Autodesk Fusion 360 part; units mm, degrees
sketch "Sketch4" plane through (0, 0, 0) normal (0, 0, 1) x (1, 0, 0)
  circle A0 centre (0, 0) radius 12.7
  dimension "d28" = 25.4
extrude "Extrude4" add sketch "Sketch4" along normal blind 25.4
sketch "Sketch5" plane through (0, 0, 25.4) normal (0, 0, 1) x (-1, 0, 0)
  circle A0 centre (0, 0) radius 12.7
  circle A1 centre (0, 0) radius 15.24
extrude "Extrude5" add sketch "Sketch5" along normal blind 5.08 contours A0 | A1
chamfer "Chamfer2" distance 2.54 angle 45 1 edges at (-11.8406, -4.5925, 0)
Verification items for the finished model (mm, model axes). A direction names the side the tool comes from. Coordinates: 2 decimals unless noted, no trailing zeros. Order: outer loops, then holes, each group sorted by start corner. A loop starts at its lowest first (then second) coordinate and runs counter-clockwise, first axis right, second up.
1. Set-up check for faces 1 (the face through (0, 0, 30.48)), 2 (the face through (3.5, -12.5, 25.4)): record each of +Z, -Z, +X, -X, +Y, -Y from which the full face is reachable in a straight line by a thin tool's end or side.
Results found:
face 1: +Z, +X, -X, +Y, -Y
face 2: -Z
2. Scan lines: line 1 (Z direction, x = 10, y = 8); line 2 (X direction, y = 0.5, z = 3); line 3 (X direction, y = 9, z = 12.5). Record each from-to range of solid material in increasing order.
Results found:
line 1: z = 25.4 to 30.48
line 2: x = -12.69 to 12.69
line 3: x = -8.96 to 8.96
3. Sectioned sample at A-A, the plane y = 0. Record the cut outline in (x, z), and give its area (3 significant figures).
Results found:
outline: (-15.24, 25.4) - (-12.7, 25.4) - (-12.7, 2.54) - (-10.16, 0) - (10.16, 0) - (12.7, 2.54) - (12.7, 25.4) - (15.24, 25.4) - (15.24, 30.48) - (-15.24, 30.48) - close
area: 794 mm2
4. Go/stop test with flat-tipped pins: pin 1 Ø4 at (y, z) = (-12, 5) entering from +X; pin 2 Ø6 at (x, z) = (-8.5, 9.5) entering from -Y; pin 3 Ø3 at (x, z) = (-2.5, 9.5) entering from +Y. Record where each tip stops, or that it passes through.
Results found:
pin 1: stops at x = 7.83
pin 2: stops at y = -11.45
pin 3: stops at y = 12.66
5. Sectioned sample at C-C, the plane z = 3. Record the cut outline in (x, y), and give its area (3 significant figures).
Results found:
outline: circle Ø25.4 at (0, 0)
area: 507 mm2
